Geometry: see drawing. Coordinates: mm, zero at the bounding-box minimum. A direction names the side the tool comes from. Give positions to 0.01 mm unless a question says otherwise; leave off trailing zeros. Order: outer loops, then holes, each group sorted by start corner. A loop starts at its lowest first (then second) coordinate and runs counter-clockwise, first axis right, second up. Notation, with made-up numbers: M -3,37.25 L 12,37.25 A29 cw 12,60.25 Z; hole C 20,11 d2. An arc over 180 degrees is marked long. Use a Markdown table: item, result.
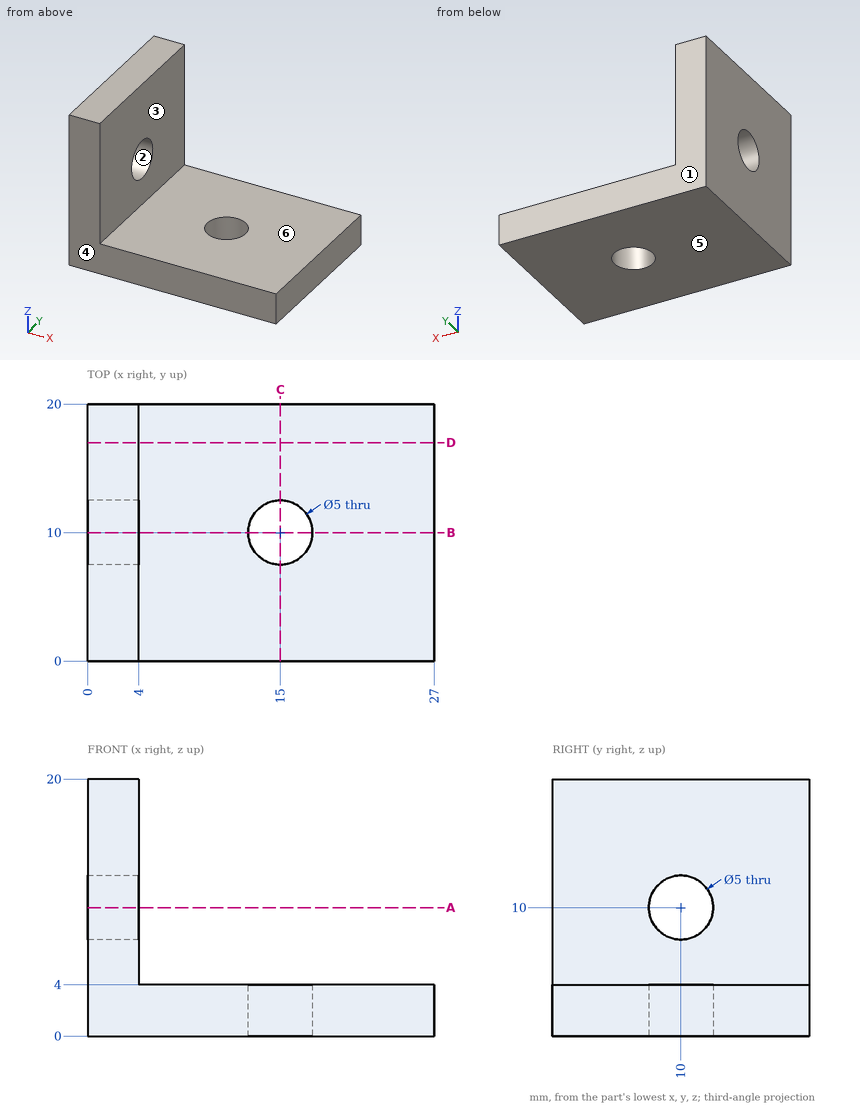
1) Material intervals for line 1 (Y direction, x = 2.85, z = 10); line 2 (X direction, y = 10, z = 2.1), sorted ascending. Write a range as from..to.
Response values:
| item | result |
|---|---|
| line 1 | y = 0..7.5, 12.5..20 |
| line 2 | x = 0..12.5, 17.5..27 |
2) Cut plane B-B on y = 10. Return loops of the section in (x, z), and give its area (3 significant figures).
Response values:
| item | result |
|---|---|
| outline | M 0,0 L 12.5,0 L 12.5,4 L 4,4 L 4,7.5 L 0,7.5 Z; M 0,12.5 L 4,12.5 L 4,20 L 0,20 Z; M 17.5,0 L 27,0 L 27,4 L 17.5,4 Z |
| area | 132 mm² |
3) Cut plane A-A on z = 10. Return loops of the section in (x, y), and give its area (3 significant figures).
Response values:
| item | result |
|---|---|
| outline | M 0,0 L 4,0 L 4,7.5 L 0,7.5 Z; M 0,12.5 L 4,12.5 L 4,20 L 0,20 Z |
| area | 60.0 mm² |
4) Cut plane D-D on y = 17. Return loops of the section in (x, z).
Response values:
| item | result |
|---|---|
| outline | M 0,0 L 27,0 L 27,4 L 4,4 L 4,20 L 0,20 Z |
5) Reachability of the marked faces 5 and 6 from +Z, -Z, +X, -X, +Y, -Y: full face, straight path, thin tool, end or side. Return the list, or none.
Response values:
| item | result |
|---|---|
| face 5 | -Z, +X, -X, +Y, -Y |
| face 6 | +Z, +X, +Y, -Y |
6) Mould query, pull axis Y, two halves, no side actions, for the marked faces 1, 2, 3 and 4. Classes: released by +Y, released by -Y, zero draft, split by the parting line, or undercut.
Response values:
| item | result |
|---|---|
| face 1 | released by +Y |
| face 2 | undercut |
| face 3 | zero draft |
| face 4 | released by -Y |
7) Cut plane C-C on x = 15. Return loops of the section in (y, z), and give its area (3 significant figures).
Response values:
| item | result |
|---|---|
| outline | M 0,0 L 7.5,0 L 7.5,4 L 0,4 Z; M 12.5,0 L 20,0 L 20,4 L 12.5,4 Z |
| area | 60.0 mm² |
8) First-contact query: pin 1 Ø12 at (x, y) = (23, 17.5) entering from +Z; pin 2 Ø10 at (x, y) = (8, 3) entering from -Z. Flat tips, straight axial feed; report the tip coordinate or a pass-through.
Response values:
| item | result |
|---|---|
| pin 1 | stops at z = 4 |
| pin 2 | stops at z = 0 |
